Geometry: final body of the model. Coordinates: model frame, mm. A direction names the side the tool comes from. Coordinates: 2 decimals unless noted, no trailing zeros. Put each result on its own line as item: value.
```python
from build123d import *

# Parameters (mm, degrees)
SKETCH1_W           = 355.6
SKETCH1_H           = 114.3
SKETCH1_R           = 2.15265
SKETCH1_W_2         = 6.35
SKETCH1_H_2         = 6.604
BOSS_EXTRUDE1_DEPTH = 6.604


with BuildPart() as part:
    # Sketch1 → Boss-Extrude1 (new body)
    with BuildSketch(Plane(origin=(0, 0, 0), x_dir=(0, 0, -1), z_dir=(1, 0, 0))):
        with Locations((0, 57.15)):
            Rectangle(SKETCH1_W, SKETCH1_H)
        with Locations((-152.4, 9.525)):
            Circle(SKETCH1_R, mode=Mode.SUBTRACT)
        with Locations((0, 9.525)):
            Circle(SKETCH1_R, mode=Mode.SUBTRACT)
        with Locations((152.4, 9.525)):
            Circle(SKETCH1_R, mode=Mode.SUBTRACT)
        with Locations((-142.875, 9.525)):
            Rectangle(SKETCH1_W_2, SKETCH1_H_2, mode=Mode.SUBTRACT)
        with Locations((-161.925, 9.525)):
            Rectangle(SKETCH1_W_2, SKETCH1_H_2, mode=Mode.SUBTRACT)
        with Locations((9.525, 9.525)):
            Rectangle(SKETCH1_W_2, SKETCH1_H_2, mode=Mode.SUBTRACT)
        with Locations((-9.525, 9.525)):
            Rectangle(SKETCH1_W_2, SKETCH1_H_2, mode=Mode.SUBTRACT)
        with Locations((161.925, 9.525)):
            Rectangle(SKETCH1_W_2, SKETCH1_H_2, mode=Mode.SUBTRACT)
        with Locations((142.875, 9.525)):
            Rectangle(SKETCH1_W_2, SKETCH1_H_2, mode=Mode.SUBTRACT)
    extrude(amount=BOSS_EXTRUDE1_DEPTH)


solid = part.part
```
1. Set-up query: faces 5 (the flat face through (3, 12.827, 143)), 6 (the flat face through (3, 56, -177.8)). Return all of +Z, -Z, +X, -X, +Y, -Y with unobstructed straight access to the full face (end or side cutting, diameter ignored); none if empty.
Answer below:
face 5: +X, -X
face 6: -Z, +X, -X, +Y, -Y
2. Mould query, pull axis Z, two halves, no side actions, for faces 1 (the flat face through (3, 56, 177.8)), 2 (the flat face through (0, 58, 2)), 3 (the flat face through (3, 9, 165.1)), 4 (the flat face through (3, 12.827, 162)). Classes: +Z half, -Z half, draft (parallel to the pull), parting line (faces both ways), or undercut.
Answer below:
face 1: +Z half
face 2: draft
face 3: undercut
face 4: undercut
3. Ray query, probe 1 along Y at (x, z) = (4.25, 0). Return the intervals inside material, ascending. Write a range as from..to.
Answer below:
probe 1: y = 0..7.37, 11.68..114.3
